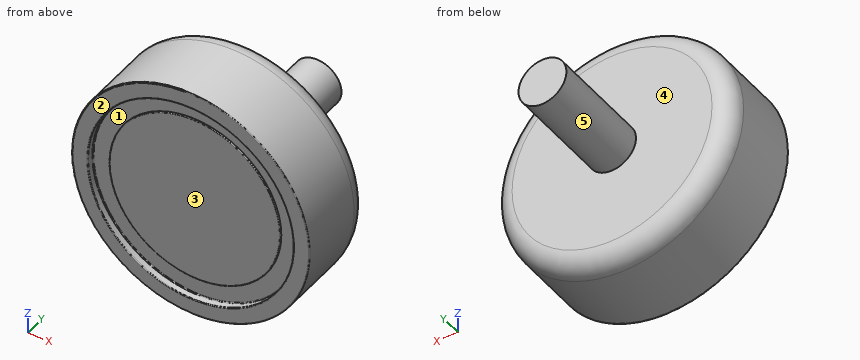
```python
from build123d import *

# Parameters (mm, degrees)
SKETCH2_R           = 1.9
BOSS_EXTRUDE1_DEPTH = 8.25
FILLET1_R           = 0.0635


with BuildPart() as part:
    # Sketch1 → Revolve1 (revolve)
    with BuildSketch(Plane.XY):
        with BuildLine():
            Line((-9.43, 0), (-8.16, 0))
            Line((-8.16, 0), (-8.16, 0.6))
            Line((-8.16, 0.6), (-6.8, 0.6))
            Line((-6.8, 0.6), (-6.8, 0.5))
            Line((-6.8, 0.5), (0, 0.5))
            Line((0, 0.5), (0, 6.8))
            Line((0, 6.8), (-7.93, 6.8))
            ThreePointArc((-7.93, 6.8), (-8.990660172, 6.360660172), (-9.43, 5.3))
            Line((-9.43, 5.3), (-9.43, 0))
        make_face()
    revolve(axis=Axis((0, 6.8, 0), (0, -1, 0)))

    # Sketch2 → Boss-Extrude1 (add)
    with BuildSketch(Plane(origin=(0, 6.8, 0), x_dir=(1, 0, 0), z_dir=(0, 1, 0))):
        Circle(SKETCH2_R)
    extrude(amount=BOSS_EXTRUDE1_DEPTH)

    # Fillet1
    fillet1_edges = [part.edges().sort_by_distance(p)[0] for p in [
        (8.16, 0.6, 0),
        (8.16, 0, 0),
        (9.43, 0, 0),
        (6.8, 0.5, 0),
    ]]
    fillet(fillet1_edges, radius=FILLET1_R)


solid = part.part
```
Source: CAD feature listing. Evaluate the final solid. Frame: model axes, mm. Face numbers are marked on the shaded views. A direction names the side the tool comes from. Round coordinates to 2 decimals unless told otherwise and drop trailing zeros. Write each loop counter-clockwise with the first axis right and the second up, starting at its lowest first coordinate (ties: lowest second). Pieces come first, ordered by that corner, then holes. Notation, with made-up numbers: M 21.5,0 L 31.5,0 A33 ccw 31.5,29 Z; hole C 43.5,32 d8. An arc over 180 degrees is marked long. Answer as a JSON object with one key per item and string values. Group by question number.
(1) Mould query, pull axis Z, two halves, no side actions, for the marked faces 3, 4 and 5. Classes: +Z half, -Z half, draft (parallel to the pull), parting line (faces both ways), or undercut.
(2) Section query C-C on y = 12.75. Output: boundary loops of the cut face in (x, z), then the cut area to 3 significant figures.
(3) Reachability of the marked faces 1 and 2 from +Z, -Z, +X, -X, +Y, -Y: full face, straight path, thin tool, end or side. Return the list, or none.
(4) Section query D-D on y = 6.5. Output: boundary loops of the cut face in (x, z), then the cut area to 3 significant figures.
(5) Ray query, line 1 (X direction, y = 0.25, z = 0); line 2 (Y direction, x = -0.25, z = -5.25). Return the intervals inside material, ascending. Write a range as [from, to].
(6) First-contact query: pin 1 (1 mm diameter, centred on y = 3.5, z = -5, fed in from +X); pin 2 (1 mm diameter, centred on y = 11.5, z = 2, fed in from +X); pin 3 (3 mm diameter, centred on x = -6.5, z = -0.5, fed in from -Y). Flat tips, straight axial feed; report the tip coordinate or a pass-through.
Computed values:
{
 "1": {"face 3": "undercut", "face 4": "draft", "face 5": "parting line"},
 "2": {"outline": "C 0,0 d3.8", "area": "11.3 mm^2"},
 "3": {"face 1": "-Y", "face 2": "+Z, -Z, +X, -X, -Y"},
 "4": {"outline": "C 0,0 d17.66", "area": "245 mm^2"},
 "5": {"line 1": "[-9.43, -8.16], [8.16, 9.43]", "line 2": "[0.5, 6.8]"},
 "6": {"pin 1": "x = 8.29", "pin 2": "x = 1.17", "pin 3": "y = 0.5"}
}
